Could you check a few things on this model? Use its own coordinates, in mm. Coordinates: 2 decimals unless noted, no trailing zeros. Order: outer loops, then holes, each group sorted by start corner. A loop starts at its lowest first (then second) coordinate and runs counter-clockwise, first axis right, second up. Notation, with made-up numbers: (20, 44) -> (48, 44) arc R26 cw to (48, 77) -> close; hole circle Ø9 at (63.25, 29). An arc over 180 degrees is marked (long way). Use a Markdown table: item, result. Add a question column.
1) Thinking about a two-plate mould opening in X: for faces 1 (the cylindrical face through (-1.938, -0.44, 1.972)), 2 (the flat face through (7.5, 0, 2)), 3 (the flat face through (0, -1.719, 2)), which applies, +X half, -X half, draft (parallel to the pull), parting line (faces both ways), or undercut?
2) If I drill on L1, parallel to X at y = -0.05, z = 0.55; L2, parallel to Y at x = 0, z = 2.9; L3, parallel to X at y = -0.3, z = 2.3, over which ranges is the centre line in solid material (lowest first)? Write a range as [from, to].
3) If we section it at B-B (x = 0): Write out the boundary of the cut face in (y, z).
4) If we section it at C-C (z = 2.9): Write out the boundary of the cut face in (x, y), plus the area to 3 significant figures.
5) If we section it at D-D (x = -6): Write out the boundary of the cut face in (y, z), plus the area to 3 significant figures.
6) If we section it at A-A (y = 0): Write out the boundary of the cut face in (x, z).
7) Will this pin go through, and if not, where does the flat tip stop? pin 1 Ø1.3 at (x, y) = (0, 0) entering from +Z (3 decimals).
```python
from build123d import *

# Parameters (mm, degrees)
SKETCH1_W           = 15
SKETCH1_H           = 3.437195072
SKETCH1_R           = 1.2
SKETCH1_R_2         = 1
SKETCH1_R_3         = 1.05
SKETCH1_R_4         = 1.15
SKETCH1_R_5         = 1.1
BOSS_EXTRUDE1_DEPTH = 4


with BuildPart() as part:
    # Sketch1 → Boss-Extrude1 (new body)
    with BuildSketch(Plane.XY):
        Rectangle(SKETCH1_W, SKETCH1_H)
        with Locations((-6, 0)):
            Circle(SKETCH1_R, mode=Mode.SUBTRACT)
        with Locations((5.536057004, 0)):
            Circle(SKETCH1_R_2, mode=Mode.SUBTRACT)
        with Locations((3, 0)):
            Circle(SKETCH1_R_3, mode=Mode.SUBTRACT)
        with Locations((-3, 0)):
            Circle(SKETCH1_R_4, mode=Mode.SUBTRACT)
        Circle(SKETCH1_R_5, mode=Mode.SUBTRACT)
    extrude(amount=BOSS_EXTRUDE1_DEPTH)


solid = part.part
```
Answer sheet:
| question | item | result |
|---|---|---|
| 1 | face 1 | undercut |
| 1 | face 2 | +X half |
| 1 | face 3 | draft |
| 2 | L1 | [-7.5, -7.2], [-4.8, -4.15], [-1.85, -1.1], [1.1, 1.95], [4.05, 4.54], [6.53, 7.5] |
| 2 | L2 | [-1.72, -1.1], [1.1, 1.72] |
| 2 | L3 | [-7.5, -7.16], [-4.84, -4.11], [-1.89, -1.06], [1.06, 1.99], [4.01, 4.58], [6.49, 7.5] |
| 3 | outline | (-1.72, 0) -> (-1.1, 0) -> (-1.1, 4) -> (-1.72, 4) -> close; (1.1, 0) -> (1.72, 0) -> (1.72, 4) -> (1.1, 4) -> close |
| 4 | outline | (-7.5, -1.72) -> (7.5, -1.72) -> (7.5, 1.72) -> (-7.5, 1.72) -> close; hole circle Ø2.4 at (-6, 0); hole circle Ø2.3 at (-3, 0); hole circle Ø2.2 at (0, 0); hole circle Ø2.1 at (3, 0); hole circle Ø2 at (5.54, 0) |
| 4 | area | 32.5 mm2 |
| 5 | outline | (-1.72, 0) -> (-1.2, 0) -> (-1.2, 4) -> (-1.72, 4) -> close; (1.2, 0) -> (1.72, 0) -> (1.72, 4) -> (1.2, 4) -> close |
| 5 | area | 4.15 mm2 |
| 6 | outline | (-7.5, 0) -> (-7.2, 0) -> (-7.2, 4) -> (-7.5, 4) -> close; (-4.8, 0) -> (-4.15, 0) -> (-4.15, 4) -> (-4.8, 4) -> close; (-1.85, 0) -> (-1.1, 0) -> (-1.1, 4) -> (-1.85, 4) -> close; (1.1, 0) -> (1.95, 0) -> (1.95, 4) -> (1.1, 4) -> close; (4.05, 0) -> (4.54, 0) -> (4.54, 4) -> (4.05, 4) -> close; (6.54, 0) -> (7.5, 0) -> (7.5, 4) -> (6.54, 4) -> close |
| 7 | pin 1 | through |
